Autodesk Inventor part; units mm, degrees
ref_plane "YZ Plane" through (0, 0, 0) normal (1, 0, 0) x (0, 1, 0)
ref_plane "XZ Plane" through (0, 0, 0) normal (0, 1, 0) x (-1, 0, 0)
ref_plane "XY Plane" through (0, 0, 0) normal (0, 0, 1) x (1, 0, 0)
sketch "Sketch1" plane through (0, 0, 0) normal (0, 0, 1) x (1, 0, 0)
  line L0 (0, 0) -> (4.5, 0)
  line L1 (6, 0) -> (6, -2.25) construction
  line L2 (7.5, -3.75) -> (13, -3.75)
  line L3 (0, 0) -> (0, 5.6294)
  arc A0 (6, -2.25) -> (7.5, -3.75) centre (7.5, -2.25) ccw
  arc A1 (6, -1.5) -> (4.5, 0) centre (4.5, -1.5) ccw
  line L4 (6, -2.25) -> (6, -1.5)
  point P0 (6, -3.75)
  dimension "d0" = 12
  dimension "d1" = 26
  dimension "d2" = 3.75
  dimension "d3" = 1.5
surface revolve "RevolutionSrf1" sketch "Sketch1" angle 360 about axis through (0, 0, 0) along (0, 1, 0) shown no curves L2 A0 L4 A1 L0 L3
thicken "Thicken2" operation add thickness 1 both sides no extend neighbours no toward (0, -1, 0) faces at (0.8521, 0, 1.2345) (5.9182, -1.3879, 0.9618) (5.9805, -2, 0.4828) (7.2922, -3.7458, 1.1851) (11.0407, -3.75, 1.037)
sketch "Sketch3" plane through (0, 0, 0) normal (0, 1, 0) x (1, 0, 0)
  circle A0 centre (0, 0) radius 4.05
  line L0 (-3.2, 2.4824) -> (-3.2, -2.4824)
  line L1 (3.2, 2.4824) -> (3.2, -2.4824)
  dimension "d16" = 8.1
  dimension "d17" = 6.4
extrude "Extrusion2" cut sketch "Sketch3" against normal through all contours L1 A0 L0
equation "\"BendRadius\" = Thickness"
equation "\"BendReliefWidth\" = Thickness"
equation "\"BendReliefDepth\" = 0.5 * Thickness"
equation "\"CornerReliefSize\" = 4 * Thickness"
equation "\"MinimumRemnant\" = 2 * Thickness"
equation "\"TransitionRadius\" = BendRadius"
equation "\"JacobiRadiusSize\" = BendRadius"
properties part number "404-08" material "Steel, Mild"
Here's how the part is built. I have some questions about the finished solid (model axes, mm). A direction names the side the tool comes from. Round coordinates to 2 decimals unless told otherwise and drop trailing zeros. Order: outer loops, then holes, each group sorted by start corner. A loop starts at its lowest first (then second) coordinate and runs counter-clockwise, first axis right, second up. Notation, with made-up numbers: (-28.75, -34.5) -> (22.25, -34.5) arc R27 ccw to (22.25, -7.5) -> close; hole circle Ø11 at (1.25, 0.25). An arc over 180 degrees is marked (long way). Return JSON: item names as keys, results as strings.
Q1. Which directions (+Z, -Z, +X, -X, +Y, -Y) give clear straight access to the entire face, cutting with the end or side of a thin tool? Please do faces 4 (the flat face through (6, -3.75, 6)), 5 (the flat face through (-3.4, -1, 0.3)), 6 (the flat face through (3.2, -0.5, 0)).
Filled sheet:
{"face 4": "+Y", "face 5": "-Y", "face 6": "+Y, -Y"}
Q2. If we section it at B-B on x = 0: List the corners of the cut face in (y, z) for me, plus the area to 3 significant figures.
Filled sheet:
{"outline": "(-4.75, -13) -> (-3.75, -13) -> (-3.75, -7.5) arc R1.5 cw to (-2.25, -6) -> (-1.5, -6) arc R1.5 ccw to (0, -4.5) -> (0, -4.05) -> (-1, -4.05) -> (-1, -4.5) arc R0.5 cw to (-1.5, -5) -> (-2.25, -5) arc R2.5 ccw to (-4.75, -7.5) -> close; (-4.75, 7.5) arc R2.5 ccw to (-2.25, 5) -> (-1.5, 5) arc R0.5 cw to (-1, 4.5) -> (-1, 4.05) -> (0, 4.05) -> (0, 4.5) arc R1.5 ccw to (-1.5, 6) -> (-2.25, 6) arc R1.5 cw to (-3.75, 7.5) -> (-3.75, 13) -> (-4.75, 13) -> close", "area": "22.8 mm^2"}
Q3. If we section it at D-D on y = -3.15: List the corners of the cut face in (x, z) for me.
Filled sheet:
{"outline": "circle Ø12.6 at (0, 0); hole circle Ø10.34 at (0, 0)"}
Q4. If we mould it in two halves opening along Z, with no side actions, what happens to faces 1 (the cylindrical face through (-1.08, -1.87, 4.88)), 2 (the cylindrical face through (-6, -2, 0)), 3 (the flat face through (-3.4, 0, 0.3))? For each: released by +Z, released by -Z, zero draft, split by the parting line, or undercut.
Filled sheet:
{"face 1": "undercut", "face 2": "split by the parting line", "face 3": "zero draft"}
Q5. I need wall thicknesses on line 1 along Z through (x, y) = (0, -1.7); line 2 along Y through (x, z) = (8.75, 1.25). Which ranges of each line are inside material? Lowest first, please. Write a range as from..to.
Filled sheet:
{"line 1": "z = -6..-5, 5..6", "line 2": "y = -4.75..-3.75"}
Q6. For pin 1 Ø9 at (x, z) = (0, 0) entering from -Y; pin 2 Ø1 at (x, y) = (2, -3) entering from +Z; pin 3 Ø8 at (x, z) = (2.5, 2.5) entering from +Y; pin 4 Ø5 at (x, z) = (10, 9.5) entering from +Y, each with a flat end and sliding along its axis, tell me the tip position at first contact or that it passes through.
Filled sheet:
{"pin 1": "stops at y = -1", "pin 2": "stops at z = 6.38", "pin 3": "stops at y = 0", "pin 4": "stops at y = -3.75"}
Q7. If we section it at C-C on y = -0.35: List the corners of the cut face in (x, z) for me.
Filled sheet:
{"outline": "circle Ø10.93 at (0, 0); hole (-3.2, -2.48) arc R4.05 ccw to (3.2, -2.48) -> (3.2, 2.48) arc R4.05 ccw to (-3.2, 2.48) -> close"}
Q8. If we section it at A-A on z = 0: List the corners of the cut face in (x, y) for me.
Filled sheet:
{"outline": "(-13, -4.75) -> (-7.5, -4.75) arc R2.5 ccw to (-5, -2.25) -> (-5, -1.5) arc R0.5 cw to (-4.5, -1) -> (-3.2, -1) -> (-3.2, 0) -> (-4.5, 0) arc R1.5 ccw to (-6, -1.5) -> (-6, -2.25) arc R1.5 cw to (-7.5, -3.75) -> (-13, -3.75) -> close; (3.2, -1) -> (4.5, -1) arc R0.5 cw to (5, -1.5) -> (5, -2.25) arc R2.5 ccw to (7.5, -4.75) -> (13, -4.75) -> (13, -3.75) -> (7.5, -3.75) arc R1.5 cw to (6, -2.25) -> (6, -1.5) arc R1.5 ccw to (4.5, 0) -> (3.2, 0) -> close"}
